from build123d import *

# Parameters (mm, degrees)
SKETCH1_R           = 50
BOSS_EXTRUDE1_DEPTH = 2
SKETCH2_R           = 47.75
BOSS_EXTRUDE2_DEPTH = 2
SKETCH3_R           = 7.25
CUT_EXTRUDE1_DEPTH  = 71.823724839


with BuildPart() as part:
    # Sketch1 → Boss-Extrude1 (new body)
    with BuildSketch(Plane(origin=(0, 0, 0), x_dir=(1, 0, 0), z_dir=(0, 1, 0))):
        with Locations(Location((0, 0, 0), (0, 0, 270))):
            Circle(SKETCH1_R)
    extrude(amount=BOSS_EXTRUDE1_DEPTH)

    # Sketch2 → Boss-Extrude2 (add)
    with BuildSketch(Plane.XZ):
        with Locations(Location((0, 0, 0), (0, 0, 270))):
            Circle(SKETCH2_R)
    extrude(amount=BOSS_EXTRUDE2_DEPTH)

    # Sketch3 → Cut-Extrude1 (cut, through all)
    with BuildSketch(Plane(origin=(0, 2, 0), x_dir=(1, 0, 0), z_dir=(0, 1, 0))):
        with Locations(Location((-20, 0, 0), (0, 0, 270))):
            Circle(SKETCH3_R)
        with Locations(Location((20, 0, 0), (0, 0, 270))):
            Circle(SKETCH3_R)
    extrude(amount=-CUT_EXTRUDE1_DEPTH, mode=Mode.SUBTRACT)


solid = part.part
Work out the finished part from the listing and answer in its coordinate system (mm). A direction names the side the tool comes from. Give positions to 0.01 mm unless a question says otherwise; leave off trailing zeros. Loops run counter-clockwise (first coordinate to the right, second up) from the corner with the lowest first, then second, coordinate; pieces in that order, holes last. Notation, with made-up numbers: (70, -12) - (84, -12) arc R31 cw to (84, 27) - close; hole circle Ø10 at (89, 51). An arc over 180 degrees is marked (long way). Answer in a Markdown table with one row per item. Add a question column.
Q1. This flat-tipped pin is pushed along its axis until it touches: P1, Ø8.5, axis at x = 20, z = 0, coming from the -Y side. Where does it stop, or does it pass through?
Q2. A tool of negligible diameter and unlimited length cuts with its end or side. For faces 1 (the flat face through (-41, 0, 26)), 2 (the cylindrical face through (15.02, 0.99, 47.69)), from which of +Z, -Z, +X, -X, +Y, -Y can it reach the whole face along a straight path? Write none if from no direction.
Q3. The part is cut by section A-A (z = 0). Determine the outline of the cut face in (x, y), and give its area (3 significant figures).
Q4. The part is cut by section D-D (x = 0). Determine the outline of the cut face in (y, z).
Q5. The part is cut by section C-C (y = 0.95). Determine the outline of the cut face in (x, z), and give its area (3 significant figures).
Q6. Consider line 1 along X through (y, z) = (0.45, 0); line 2 along X through (y, z) = (-0.2, 0); line 3 along Y through (x, z) = (-23.5, 43.5). Determine where each line is inside the solid, lowest interval first.
Q7. The part is cut by section B-B (x = -20). Determine the outline of the cut face in (y, z), and give its area (3 significant figures).
Q8. Determine the mould class of faces 3 (the cylindrical face through (26.11, 0.03, 3.9)), 4 (the flat face through (1, -2, 1)), 5 (the cylindrical face through (-13.89, 0.03, 3.9)), 6 (the cylindrical face through (-46.615, -0.986, 10.351)) for opening direction X: released by +X, released by -X, zero draft, split by the parting line, or undercut.
Solution:
| question | item | result |
|---|---|---|
| 1 | P1 | passes through |
| 2 | face 1 | -Y |
| 2 | face 2 | +Y, -Y |
| 3 | outline | (-50, 0) - (-47.75, 0) - (-47.75, -2) - (-27.25, -2) - (-27.25, 2) - (-50, 2) - close; (-12.75, -2) - (12.75, -2) - (12.75, 2) - (-12.75, 2) - close; (27.25, -2) - (47.75, -2) - (47.75, 0) - (50, 0) - (50, 2) - (27.25, 2) - close |
| 3 | area | 275 mm² |
| 4 | outline | (-2, -47.75) - (0, -47.75) - (0, -50) - (2, -50) - (2, 50) - (0, 50) - (0, 47.75) - (-2, 47.75) - close |
| 5 | outline | circle Ø100 at (0, 0); hole circle Ø14.5 at (-20, 0); hole circle Ø14.5 at (20, 0) |
| 5 | area | 7,520 mm² |
| 6 | line 1 | x = -50 to -27.25, -12.75 to 12.75, 27.25 to 50 |
| 6 | line 2 | x = -47.75 to -27.25, -12.75 to 12.75, 27.25 to 47.75 |
| 6 | line 3 | y = 0 to 2 |
| 7 | outline | (-2, -43.36) - (0, -43.36) - (0, -45.83) - (2, -45.83) - (2, -7.25) - (-2, -7.25) - close; (-2, 7.25) - (2, 7.25) - (2, 45.83) - (0, 45.83) - (0, 43.36) - (-2, 43.36) - close |
| 7 | area | 299 mm² |
| 8 | face 3 | undercut |
| 8 | face 4 | zero draft |
| 8 | face 5 | undercut |
| 8 | face 6 | split by the parting line |
